The listing builds one solid part. Answer for the finished solid, in the listing's coordinates (mm). A direction names the side the tool comes from. Give positions to 0.01 mm unless a question says otherwise; leave off trailing zeros. Order: outer loops, then holes, each group sorted by start corner. A loop starts at its lowest first (then second) coordinate and runs counter-clockwise, first axis right, second up. Notation, with made-up numbers: (20, 14) - (43, 14) arc R26 ccw to (43, 50) - close; hole circle Ø4 at (10, 5). An arc over 180 degrees is marked (long way). Answer as CSV lines item,"result". Start each with the question number.
1. Section C-C on x = 179.5 is taken. Give the vertices of the cut face in (y, z), and give its area (3 significant figures).
2. Section B-B on z = -9 is taken. Give the vertices of the cut face in (x, y), and give its area (3 significant figures).
3. Flat-ended cylindrical pins translate along their axes: pin 1 (8 mm diameter, centred on x = 175, y = -11.5, fed in from -Z); pin 2 (0.5 mm diameter, centred on y = -7, z = 0.5, fed in from -X); pin 3 (0.8 mm diameter, centred on y = 1.5, z = 1, fed in from +X). Find the tip coordinate at first contact, or state that the pin passes through.
4. Section A-A on y = -35 is taken. Give the vertices of the cut face in (x, z).
5. Consider line 1 along X through (y, z) = (33.5, -29.5); line 2 along Z through (x, y) = (206, 49.5); line 3 along X through (y, z) = (-33, -1). Determine where each line is inside the solid, lowest interval first. Write a range as [from, to].
6. Which of the six approach directions +Z, -Z, +X, -X, +Y, -Y give full straight-line access (tool end or side, diameter ignored) to faces 4 (the flat face through (-257.2, -1, -19)), 5 (the flat face through (-257.989, -49.566, -18.806))?
7. Determine the mould class of faces 1 (the flat face through (258.801, 1, -19)), 2 (the flat face through (1, 59.5, 1)), 3 (the flat face through (-4, -12, 0)) for opening direction X: +X half, -X half, draft (parallel to the pull), parting line (faces both ways), or undercut.
from build123d import *

# Parameters (mm, degrees)
SKETCH1_W                      = 514.4008
SKETCH1_H                      = 119
BOSS_EXTRUDE1_DEPTH            = 1.6002
EDGE_FLANGE1_STRIP_W           = 9.6012
EDGE_FLANGE1_STRIP_H           = 1.6002
EDGE_FLANGE1_STRIP_CUT_DEPTH   = 119
EDGE_FLANGE1_STRIP_2_W         = 9.6012
EDGE_FLANGE1_STRIP_2_H         = 1.6002
EDGE_FLANGE1_STRIP_CUT_2_DEPTH = 119
EDGE_FLANGE1_DEPTH             = 119
EDGE_FLANGE1_BEND_DEPTH        = 119
SKETCH19_R                     = 3.2639
CUT_EXTRUDE1_DEPTH             = 523.286786777
SKETCH21_R                     = 1.25
SKETCH21_W                     = 117.999999966
SKETCH21_H                     = 53
CUT_EXTRUDE3_DEPTH             = 2.54
SKETCH22_W                     = 21.9964
SKETCH22_H                     = 30.2006
CUT_EXTRUDE4_DEPTH             = 2.54
SKETCH23_R                     = 1.079501479
SKETCH23_W                     = 69.208094806
SKETCH23_H                     = 27.008036997
CUT_EXTRUDE5_DEPTH             = 2.54
CHAMFER1_SIZE                  = 0.5
CUT_EXTRUDE6_DEPTH             = 523.286786777


# Sheet-metal steps are written as plain solids
with BuildPart() as part:
    # Sketch1 → Boss-Extrude1 (new body)
    with BuildSketch(Plane.XY):
        Rectangle(SKETCH1_W, SKETCH1_H)
    extrude(amount=BOSS_EXTRUDE1_DEPTH)

    # Edge-Flange1 strip (across the edge) → Edge-Flange1 strip cut (cut)
    with BuildSketch(Plane(origin=(257.2004, 59.5, 0), x_dir=(-1, 0, 0), z_dir=(0, -1, 0))):
        with Locations((-3.2004, -0.8001)):
            Rectangle(EDGE_FLANGE1_STRIP_W, EDGE_FLANGE1_STRIP_H)
    extrude(amount=EDGE_FLANGE1_STRIP_CUT_DEPTH, mode=Mode.SUBTRACT)

    # Edge-Flange1 strip 2 (across the edge) → Edge-Flange1 strip cut 2 (cut)
    with BuildSketch(Plane(origin=(-257.2004, -59.5, 0), x_dir=(1, 0, 0), z_dir=(0, 1, 0))):
        with Locations((-3.2004, -0.8001)):
            Rectangle(EDGE_FLANGE1_STRIP_2_W, EDGE_FLANGE1_STRIP_2_H)
    extrude(amount=EDGE_FLANGE1_STRIP_CUT_2_DEPTH, mode=Mode.SUBTRACT)

    # Edge-Flange1 section (across the edge) → Edge-Flange1 (add)
    with BuildSketch(Plane(origin=(257.2004, 59.5, 0), x_dir=(-1, 0, 0), z_dir=(0, -1, 0))):
        with BuildLine():
            Line((-1.6002, 1.6002), (-1.6002, 36.4998))
            Line((-1.6002, 36.4998), (0, 36.4998))
            Line((0, 36.4998), (0, 1.6002))
            ThreePointArc((0, 1.6002), (0.468687729, 0.468687729), (1.6002, 0))
            Line((1.6002, 0), (1.6002, -1.6002))
            ThreePointArc((1.6002, -1.6002), (-0.662824543, -0.662824543), (-1.6002, 1.6002))
        make_face()
    extrude(amount=EDGE_FLANGE1_DEPTH)

    # Edge-Flange1 section 2 (across the edge) → Edge-Flange1 bend (add)
    with BuildSketch(Plane(origin=(-257.2004, -59.5, 0), x_dir=(1, 0, 0), z_dir=(0, 1, 0))):
        with BuildLine():
            Line((-1.6002, 1.6002), (-1.6002, 36.4998))
            Line((-1.6002, 36.4998), (0, 36.4998))
            Line((0, 36.4998), (0, 1.6002))
            ThreePointArc((0, 1.6002), (0.468687729, 0.468687729), (1.6002, 0))
            Line((1.6002, 0), (1.6002, -1.6002))
            ThreePointArc((1.6002, -1.6002), (-0.662824543, -0.662824543), (-1.6002, 1.6002))
        make_face()
    extrude(amount=EDGE_FLANGE1_BEND_DEPTH)

    # Sketch19 → Cut-Extrude1 (cut, through all)
    with BuildSketch(Plane(origin=(258.8006, 0, 0), x_dir=(0, 0, -1), z_dir=(1, 0, 0))):
        with Locations((17.4498, 21.4)):
            Circle(SKETCH19_R)
        with Locations((17.4498, -16.7)):
            Circle(SKETCH19_R)
    extrude(amount=-CUT_EXTRUDE1_DEPTH, mode=Mode.SUBTRACT)

    # Sketch21 → Cut-Extrude3 (cut)
    with BuildSketch(Plane.XY.offset(1.6002)):
        with Locations((-204.299799983, 32.869379504)):
            Circle(SKETCH21_R)
        with Locations((-80.299799983, 32.869379504)):
            Circle(SKETCH21_R)
        with Locations((-204.299799983, -24.130620496)):
            Circle(SKETCH21_R)
        with Locations((-80.299799983, -24.130620496)):
            Circle(SKETCH21_R)
        with Locations((-138.0998, 4.619379504)):
            Rectangle(SKETCH21_W, SKETCH21_H)
    extrude(amount=-CUT_EXTRUDE3_DEPTH, mode=Mode.SUBTRACT)

    # Sketch22 → Cut-Extrude4 (cut)
    with BuildSketch(Plane.XY.offset(1.6002)):
        with Locations((201.5998, 4.619379504)):
            Rectangle(SKETCH22_W, SKETCH22_H)
    extrude(amount=-CUT_EXTRUDE4_DEPTH, mode=Mode.SUBTRACT)

    # Sketch23 → Cut-Extrude5 (cut)
    with BuildSketch(Plane.XY.offset(1.6002)):
        with Locations((-16.92801633, 19.475664516)):
            Circle(SKETCH23_R)
        with Locations((-16.92801633, -10.52437658)):
            Circle(SKETCH23_R)
        with Locations((58.07208641, 19.475664516)):
            Circle(SKETCH23_R)
        with Locations((88.572128191, 19.475664516)):
            Circle(SKETCH23_R)
        with Locations((88.572128191, -10.52437658)):
            Circle(SKETCH23_R)
        with Locations((20.57203504, 4.475643969)):
            Rectangle(SKETCH23_W, SKETCH23_H)
        with BuildLine():
            Line((81.870702539, 5.275383569), (79.720177643, 7.425908465))
            ThreePointArc((79.720177643, 7.425908465), (79.4750071, 8.658464018), (80.519917243, 9.356650655))
            Line((80.519917243, 9.356650655), (85.103371505, 9.356650655))
            ThreePointArc((85.103371505, 9.356650655), (85.537484246, 9.270020118), (85.905094187, 9.023399655))
            Line((85.905094187, 9.023399655), (89.636523764, 5.273395558))
            ThreePointArc((89.636523764, 5.273395558), (89.965803671, 4.475643968), (89.636523764, 3.677892379))
            Line((89.636523764, 3.677892379), (85.905094187, -0.072111718))
            ThreePointArc((85.905094187, -0.072111718), (85.537484246, -0.318732182), (85.103371505, -0.405362718))
            Line((85.103371505, -0.405362718), (80.519917243, -0.405362718))
            ThreePointArc((80.519917243, -0.405362718), (79.4750071, 0.292823919), (79.720177643, 1.525379472))
            Line((79.720177643, 1.525379472), (81.870702539, 3.675904368))
            ThreePointArc((81.870702539, 3.675904368), (82.201965528, 4.475643968), (81.870702539, 5.275383569))
        make_face()
        with BuildLine():
            Line((73.871846558, 9.714604607), (78.311067597, 5.275383569))
            ThreePointArc((78.311067597, 5.275383569), (78.642330586, 4.475643968), (78.311067597, 3.675904368))
            Line((78.311067597, 3.675904368), (73.871846558, -0.763316671))
            ThreePointArc((73.871846558, -0.763316671), (73.072106958, -1.094579659), (72.272367358, -0.763316671))
            Line((72.272367358, -0.763316671), (67.833146319, 3.675904368))
            ThreePointArc((67.833146319, 3.675904368), (67.50188333, 4.475643968), (67.833146319, 5.275383569))
            Line((67.833146319, 5.275383569), (72.272367358, 9.714604607))
            ThreePointArc((72.272367358, 9.714604607), (73.072106958, 10.045867596), (73.871846558, 9.714604607))
        make_face()
        with BuildLine():
            Line((72.272367358, 13.274239549), (70.121842461, 11.123714653))
            ThreePointArc((70.121842461, 11.123714653), (68.889286908, 10.87854411), (68.191100272, 11.923454253))
            Line((68.191100272, 11.923454253), (68.191100272, 16.506908516))
            ThreePointArc((68.191100272, 16.506908516), (68.277730808, 16.941021257), (68.524351272, 17.308631198))
            Line((68.524351272, 17.308631198), (72.274355369, 21.040060774))
            ThreePointArc((72.274355369, 21.040060774), (73.072106958, 21.369340682), (73.869858547, 21.040060774))
            Line((73.869858547, 21.040060774), (77.619862644, 17.308631198))
            ThreePointArc((77.619862644, 17.308631198), (77.866483108, 16.941021257), (77.953113644, 16.506908516))
            Line((77.953113644, 16.506908516), (77.953113644, 11.923454254))
            ThreePointArc((77.953113644, 11.923454254), (77.254927008, 10.87854411), (76.022371455, 11.123714653))
            Line((76.022371455, 11.123714653), (73.871846558, 13.274239549))
            ThreePointArc((73.871846558, 13.274239549), (73.072106958, 13.605502538), (72.272367358, 13.274239549))
        make_face()
        with BuildLine():
            Line((64.273511377, 3.675904368), (66.424036273, 1.525379472))
            ThreePointArc((66.424036273, 1.525379472), (66.669206816, 0.292823919), (65.624296673, -0.405362718))
            Line((65.624296673, -0.405362718), (61.040842411, -0.405362718))
            ThreePointArc((61.040842411, -0.405362718), (60.60672967, -0.318732182), (60.239119729, -0.072111718))
            Line((60.239119729, -0.072111718), (56.507690152, 3.677892379))
            ThreePointArc((56.507690152, 3.677892379), (56.178410245, 4.475643968), (56.507690152, 5.273395558))
            Line((56.507690152, 5.273395558), (60.239119729, 9.023399655))
            ThreePointArc((60.239119729, 9.023399655), (60.60672967, 9.270020118), (61.040842411, 9.356650655))
            Line((61.040842411, 9.356650655), (65.624296673, 9.356650655))
            ThreePointArc((65.624296673, 9.356650655), (66.669206816, 8.658464018), (66.424036273, 7.425908465))
            Line((66.424036273, 7.425908465), (64.273511377, 5.275383569))
            ThreePointArc((64.273511377, 5.275383569), (63.942248388, 4.475643968), (64.273511377, 3.675904368))
        make_face()
        with BuildLine():
            Line((73.871846558, -4.322951612), (76.022371455, -2.172426716))
            ThreePointArc((76.022371455, -2.172426716), (77.254927008, -1.927256173), (77.953113644, -2.972166317))
            Line((77.953113644, -2.972166317), (77.953113644, -7.555620579))
            ThreePointArc((77.953113644, -7.555620579), (77.866483108, -7.98973332), (77.619862644, -8.357343261))
            Line((77.619862644, -8.357343261), (73.869858547, -12.088772838))
            ThreePointArc((73.869858547, -12.088772838), (73.072106958, -12.418052745), (72.274355369, -12.088772838))
            Line((72.274355369, -12.088772838), (68.524351272, -8.357343261))
            ThreePointArc((68.524351272, -8.357343261), (68.277730808, -7.98973332), (68.191100272, -7.555620579))
            Line((68.191100272, -7.555620579), (68.191100272, -2.972166317))
            ThreePointArc((68.191100272, -2.972166317), (68.889286908, -1.927256173), (70.121842461, -2.172426716))
            Line((70.121842461, -2.172426716), (72.272367358, -4.322951612))
            ThreePointArc((72.272367358, -4.322951612), (73.072106958, -4.654214601), (73.871846558, -4.322951612))
        make_face()
        with BuildLine():
            Line((65.627833205, -5.059889025), (63.536573965, -2.968629784))
            ThreePointArc((63.536573965, -2.968629784), (63.169650317, -2.723459241), (62.736834364, -2.637366795))
            Line((62.736834364, -2.637366795), (59.779347184, -2.637366795))
            ThreePointArc((59.779347184, -2.637366795), (59.346531231, -2.723459241), (58.979607584, -2.968629784))
            Line((58.979607584, -2.968629784), (56.888348343, -5.059889025))
            ThreePointArc((56.888348343, -5.059889025), (56.6431778, -5.426812672), (56.557085355, -5.859628625))
            Line((56.557085355, -5.859628625), (56.557085355, -8.817115805))
            ThreePointArc((56.557085355, -8.817115805), (56.6431778, -9.249931758), (56.888348343, -9.616855406))
            Line((56.888348343, -9.616855406), (58.979607584, -11.708114646))
            ThreePointArc((58.979607584, -11.708114646), (59.346531231, -11.953285189), (59.779347184, -12.039377635))
            Line((59.779347184, -12.039377635), (62.736834364, -12.039377635))
            ThreePointArc((62.736834364, -12.039377635), (63.169650317, -11.953285189), (63.536573965, -11.708114646))
            Line((63.536573965, -11.708114646), (65.627833205, -9.616855406))
            ThreePointArc((65.627833205, -9.616855406), (65.873003748, -9.249931758), (65.959096194, -8.817115805))
            Line((65.959096194, -8.817115805), (65.959096194, -5.859628625))
            ThreePointArc((65.959096194, -5.859628625), (65.873003748, -5.426812672), (65.627833205, -5.059889025))
        make_face()
    extrude(amount=-CUT_EXTRUDE5_DEPTH, mode=Mode.SUBTRACT)

    # Chamfer1
    chamfer1_edges = [part.edges().sort_by_distance(p)[0] for p in [
        (-14.032012363, -9.02837453, 0.8001),
        (-14.032012363, 17.979662467, 0.8001),
        (55.176082443, 17.979662467, 0.8001),
        (55.176082443, -9.02837453, 0.8001),
    ]]
    chamfer(chamfer1_edges, length=CHAMFER1_SIZE)

    # Sketch24 → Cut-Extrude6 (cut, through all)
    with BuildSketch(Plane(origin=(258.8006, 0, 0), x_dir=(0, 0, -1), z_dir=(1, 0, 0))):
        Polygon((1.6002, -59.5), (36.4998, -39.350706545), (36.4998, -59.5), align=None)
    extrude(amount=-CUT_EXTRUDE6_DEPTH, mode=Mode.SUBTRACT)


solid = part.part
Checks:
1,outline,"(-59.5, 0) - (59.5, 0) - (59.5, 1.6) - (-59.5, 1.6) - close"
1,area,"190 mm²"
2,outline,"(-258.8, -55.23) - (-257.2, -55.23) - (-257.2, 59.5) - (-258.8, 59.5) - close; (257.2, -55.23) - (258.8, -55.23) - (258.8, 59.5) - (257.2, 59.5) - close"
2,area,"367 mm²"
3,pin 1,"stops at z = 0"
3,pin 2,"stops at x = -258.21"
3,pin 3,"stops at x = 257.92"
4,outline,"(-258.8, -36.5) - (-257.2, -36.5) - (-257.2, -1.6) arc R1.6 cw to (-255.6, 0) - (255.6, 0) arc R1.6 cw to (257.2, -1.6) - (257.2, -36.5) - (258.8, -36.5) - (258.8, -1.6) arc R3.2 ccw to (255.6, 1.6) - (-255.6, 1.6) arc R3.2 ccw to (-258.8, -1.6) - close"
5,line 1,"x = [-258.8, -257.2], [257.2, 258.8]"
5,line 2,"z = [0, 1.6]"
5,line 3,"x = [-258.74, -257.08], [257.08, 258.74]"
6,face 4,"-Z, +Y, -Y"
6,face 5,"-Z, +X, -X, -Y"
7,face 1,"+X half"
7,face 2,"draft"
7,face 3,"undercut"
